Read the model definition and answer for the solid it produces. Units are mm, in the model's axes. A direction names the side the tool comes from. Give positions to 0.01 mm unless a question says otherwise; leave off trailing zeros. Order: outer loops, then holes, each group sorted by start corner. A loop starts at its lowest first (then second) coordinate and runs counter-clockwise, first axis right, second up. Notation, with made-up numbers: (19, 47) - (52, 47) arc R26 ccw to (52, 79) - close; hole circle Ø1 at (13, 56.25). An arc over 180 degrees is marked (long way). Write each question's results on one line, items separated by ' | '.
from build123d import *

# Parameters (mm, degrees)
SKIZZE1_W                       = 200
SKIZZE1_H                       = 120
AUFSATZ_LINEAR_AUSTRAGEN1_DEPTH = 130
SKIZZE2_R                       = 20
AUFSATZ_LINEAR_AUSTRAGEN2_DEPTH = 360
VERRUNDUNG1_R                   = 30


with BuildPart() as part:
    # Skizze1 → Aufsatz-Linear austragen1 (new body)
    with BuildSketch(Plane.XY):
        Rectangle(SKIZZE1_W, SKIZZE1_H)
    extrude(amount=AUFSATZ_LINEAR_AUSTRAGEN1_DEPTH)

    # Skizze2 → Aufsatz-Linear austragen2 (add)
    with BuildSketch(Plane.XY.offset(130)):
        with Locations(Location((0, 0, 0), (0, 0, 180))):
            Circle(SKIZZE2_R)
    extrude(amount=AUFSATZ_LINEAR_AUSTRAGEN2_DEPTH)

    # Verrundung1
    verrundung1_edges = [part.edges().sort_by_distance(p)[0] for p in [
        (-100, 60, 65),
        (100, 60, 65),
    ]]
    fillet(verrundung1_edges, radius=VERRUNDUNG1_R)


solid = part.part
(1) Section A-A (x = 0) is taken. Give the vertices of the cut face in (y, z).
Conclusion:
outline: (-60, 0) - (60, 0) - (60, 130) - (20, 130) - (20, 490) - (-20, 490) - (-20, 130) - (-60, 130) - close
(2) Section B-B (y = 0) is taken. Give the vertices of the cut face in (x, z).
Conclusion:
outline: (-100, 0) - (100, 0) - (100, 130) - (20, 130) - (20, 490) - (-20, 490) - (-20, 130) - (-100, 130) - close
(3) Section C-C (z = 51) is taken. Give the vertices of the cut face in (x, y).
Conclusion:
outline: (-100, -60) - (100, -60) - (100, 30) arc R30 ccw to (70, 60) - (-70, 60) arc R30 ccw to (-100, 30) - close
(4) Each of these flat-tipped pins is pushed along its axis until it touches: pin 1 (6 mm diameter, centred on y = 7.5, z = 366.5, fed in from +X); pin 2 (12 mm diameter, centred on y = 27.5, z = 364.5, fed in from -X); pin 3 (3 mm diameter, centred on y = -15, z = 186, fed in from -X). Where does it stop, or does it pass through?
Conclusion:
pin 1: x = 19.49 | pin 2: through | pin 3: x = -14.76
(5) Section D-D (z = 290.5) is taken. Give the vertices of the cut face in (x, y).
Conclusion:
outline: circle Ø40 at (0, 0)
(6) The mould has two halves that part along Z. Classify faces 1 (the face through (-1, 1, 0)), 2 (the face through (90.979, 51.445, 65.91)), 3 (the face through (0, 0, 490)): pulls with the +Z half, pulls with the -Z half, needs draft (parallel to the pull), parting line crosses it, or undercut.
Conclusion:
face 1: pulls with the -Z half | face 2: needs draft | face 3: pulls with the +Z half
(7) Consider probe 1 along Z at (x, y) = (-84.5, 45); probe 2 along X at (y, z) = (1, 425.5); probe 3 along X at (y, z) = (43, 39). Determine where each line is inside the solid, lowest interval first. Write a range as [from, to].
Conclusion:
probe 1: [0, 130] | probe 2: [-19.97, 19.97] | probe 3: [-97.04, 97.04]
(8) For faces 4 (the face through (19.98, -0.88, 307.48)), 5 (the face through (-91.445, 50.979, 65.91)), determine the directions among +Z, -Z, +X, -X, +Y, -Y from which every point of the face is accessible in a straight line to the end or side of a thin tool.
Conclusion:
face 4: +Z | face 5: +Z, -Z, -X, +Y
